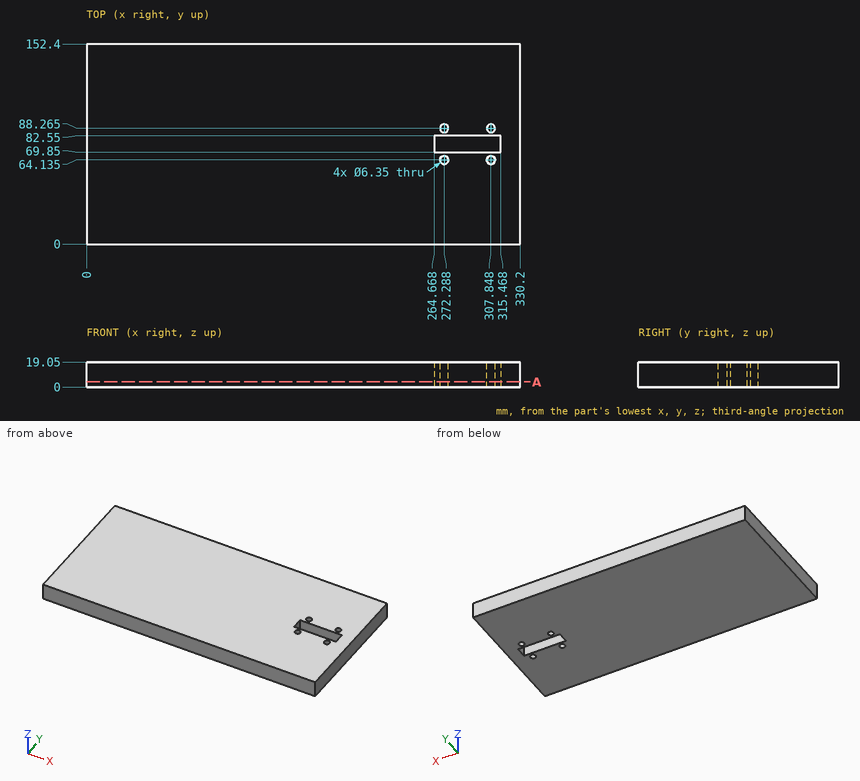
Part print with two shaded views. Sizes in mm from the minimum x, y, z corner. Round coordinates to 2 decimals unless told otherwise and drop trailing zeros. Order: outer loops, then holes, each group sorted by start corner. A loop starts at its lowest first (then second) coordinate and runs counter-clockwise, first axis right, second up. Notation, with made-up numbers: M -4.75,58.25 L 20.25,58.25 A10 ccw 20.25,63.25 Z; hole C 76,35 d4. An arc over 180 degrees is marked long. Put each result on its own line as item: value. Start each with the question number.
1. Slice it at A-A on z = 4. List the corners of the cut face in (x, y) (3 decimals), then the cut area to 3 significant figures.
2. Drill centre lines: probe 1 along X at (y, z) = (89, 1.25); probe 2 along X at (y, z) = (79.5, 6); probe 3 along Y at (x, z) = (312, 11.25). Where is each one in solid material? Low to high. Write a range as [from, to].
3. Drop a flat-ended pin along its axis: pin 1 (5 mm diameter, centred on x = 307.848, y = 64.135, fed in from +Z). Give the stop position or say it passes through.
Findings:
1. outline: M 0,0 L 330.2,0 L 330.2,152.4 L 0,152.4 Z; hole M 264.668,69.85 L 315.468,69.85 L 315.468,82.55 L 264.668,82.55 Z; hole C 272.288,64.135 d6.35; hole C 272.288,88.265 d6.35; hole C 307.848,64.135 d6.35; hole C 307.848,88.265 d6.35
1. area: 49,600 mm2
2. probe 1: [0, 269.2], [275.38, 304.76], [310.94, 330.2]
2. probe 2: [0, 264.67], [315.47, 330.2]
2. probe 3: [0, 69.85], [82.55, 152.4]
3. pin 1: through
